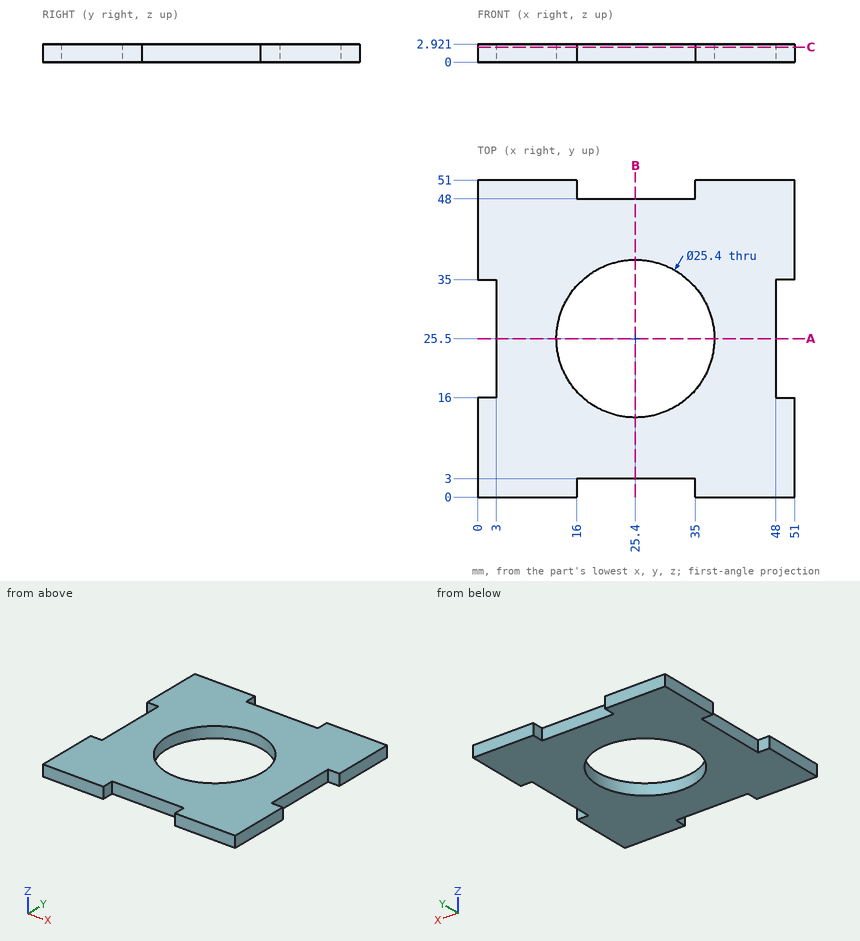
Can you work these out from the drawing? Everything is in mm from the part's minimum corner. Round coordinates to 2 decimals unless told otherwise and drop trailing zeros. Write each loop counter-clockwise with the first axis right and the second up, starting at its lowest first coordinate (ties: lowest second). Pieces come first, ordered by that corner, then holes. Notation, with made-up numbers: (-12.5, 34) - (-6.5, 34) arc R14 cw to (-6.5, 46) - close; hole circle Ø1 at (40.5, 5.25). An arc over 180 degrees is marked (long way). Write each question's results on one line, items separated by ' | '. Start each with the question number.
1) Please list where these lines run through material, in increasing order: line 1 (Y direction, x = 25.4, z = 1.2); line 2 (X direction, y = 25.5, z = 2.3); line 3 (X direction, y = 33, z = 0.1).
2) For pin 1 Ø5 at (x, y) = (38, 26.5) entering from +Z; pin 2 Ø23 at (x, y) = (25.4, 25.5) entering from -Z, each with a flat end and sliding along its axis, tell me the tip position at first contact or that it passes through.
3) Suppose I cut it at A-A (y = 25.5). List the corners of the cut face in (x, z) for me.
4) Suppose I cut it at B-B (x = 25.4). List the corners of the cut face in (y, z) for me.
5) Suppose I cut it at C-C (z = 2.4). List the corners of the cut face in (x, y) for me.
Here are the results:
1) line 1: y = 3 to 12.8, 38.2 to 48 | line 2: x = 3 to 12.7, 38.1 to 48 | line 3: x = 3 to 15.15, 35.65 to 48
2) pin 1: stops at z = 2.92 | pin 2: passes through
3) outline: (3, 0) - (12.7, 0) - (12.7, 2.92) - (3, 2.92) - close; (38.1, 0) - (48, 0) - (48, 2.92) - (38.1, 2.92) - close
4) outline: (3, 0) - (12.8, 0) - (12.8, 2.92) - (3, 2.92) - close; (38.2, 0) - (48, 0) - (48, 2.92) - (38.2, 2.92) - close
5) outline: (0, 0) - (16, 0) - (16, 3) - (35, 3) - (35, 0) - (51, 0) - (51, 16) - (48, 16) - (48, 35) - (51, 35) - (51, 51) - (35, 51) - (35, 48) - (16, 48) - (16, 51) - (0, 51) - (0, 35) - (3, 35) - (3, 16) - (0, 16) - close; hole circle Ø25.4 at (25.4, 25.5)
